```python
from build123d import *

# Parameters (mm, degrees)
ESBO_O1_R                = 7.65
ESBO_O1_R_2              = 1.65
RESSALTO_EXTRUS_O1_DEPTH = 3
FILETE1_R                = 8


with BuildPart() as part:
    # Esboço1 → Ressalto-extrusão1 (new body)
    with BuildSketch(Plane.XY):
        Polygon((-12.827454307, 0), (-5.233177242, 16.48), (5.233177242, 16.48), (12.827454307, 0), (5.233177242, -16.48), (-5.233177242, -16.48), align=None)
        Circle(ESBO_O1_R, mode=Mode.SUBTRACT)
        with Locations((0, -13.5)):
            Circle(ESBO_O1_R_2, mode=Mode.SUBTRACT)
        with Locations((0, 13.5)):
            Circle(ESBO_O1_R_2, mode=Mode.SUBTRACT)
    extrude(amount=RESSALTO_EXTRUS_O1_DEPTH)

    # Filete1
    filete1_edges = [part.edges().sort_by_distance(p)[0] for p in [
        (5.233177242, -16.48, 1.5),
        (-5.233177242, -16.48, 1.5),
        (-12.827454307, 0, 1.5),
        (-5.233177242, 16.48, 1.5),
        (5.233177242, 16.48, 1.5),
        (12.827454307, 0, 1.5),
    ]]
    fillet(filete1_edges, radius=FILETE1_R)


solid = part.part
```
Could you check a few things on this model? Use its own coordinates, in mm. Round coordinates to 2 decimals unless told otherwise and drop trailing zeros. Loops run counter-clockwise (first coordinate to the right, second up) from the corner with the lowest first, then second, coordinate; pieces in that order, holes last. Notation, with made-up numbers: (75.25, 27) - (115.25, 27) arc R26 cw to (115.25, 49) - close; hole circle Ø4 at (54.5, 83). An arc over 180 degrees is marked (long way). Answer as CSV lines item,"result".
1. I want a section at C-C on x = 4. List the corners of the cut face in (y, z) for me, then the cut area to 3 significant figures.
Filled in:
outline,"(-15.47, 0) - (-6.52, 0) - (-6.52, 3) - (-15.47, 3) - close; (6.52, 0) - (15.47, 0) - (15.47, 3) - (6.52, 3) - close"
area,"53.7 mm^2"
2. I want a section at D-D on y = 9. List the corners of the cut face in (x, z) for me, then the cut area to 3 significant figures.
Filled in:
outline,"(-8.68, 0) - (8.68, 0) - (8.68, 3) - (-8.68, 3) - close"
area,"52.1 mm^2"
3. Please list where these lines run through material, in increasing order: line 1 along Y through (x, z) = (0, 0.7); line 2 along Y through (x, z) = (-1.5, 2.85); line 3 along Y through (x, z) = (3, 2.2). Write a range as [from, to].
Filled in:
line 1,"y = [-16.48, -15.15], [-11.85, -7.65], [7.65, 11.85], [15.15, 16.48]"
line 2,"y = [-16.36, -14.19], [-12.81, -7.5], [7.5, 12.81], [14.19, 16.36]"
line 3,"y = [-15.94, -7.04], [7.04, 15.94]"
4. For pin 1 Ø1 at (y, z) = (12.5, 2.5) entering from -X; pin 2 Ø1 at (y, z) = (-11.5, 1) entering from -X, each with a flat end and sliding along its axis, tell me the tip position at first contact or that it passes through.
Filled in:
pin 1,"stops at x = -7.3"
pin 2,"stops at x = -7.76"
5. I want a section at B-B on z = 1.6. List the corners of the cut face in (x, y) for me, then the cut area to 3 significant figures.
Filled in:
outline,"(-11.28, -3.35) - (-7.38, -11.83) arc R8 ccw to (-0.11, -16.48) - (0.11, -16.48) arc R8 ccw to (7.38, -11.83) - (11.28, -3.35) arc R8 ccw to (11.28, 3.35) - (7.38, 11.83) arc R8 ccw to (0.11, 16.48) - (-0.11, 16.48) arc R8 ccw to (-7.38, 11.83) - (-11.28, 3.35) arc R8 ccw to start; hole circle Ø15.3 at (0, 0); hole circle Ø3.3 at (0, -13.5); hole circle Ø3.3 at (0, 13.5)"
area,"372 mm^2"
6. We'd pull the mould along X, two halves only. Please class faces 1 (the face through (-4.48, 15.18, 1.52)), 2 (the face through (-8, 0, 3)), 3 (the face through (-1.658, -7.468, 1.479)), 4 (the face through (12.02, 0.05, 1.52)): +X half, -X half, draft (parallel to the pull), parting line (faces both ways), or undercut.
Filled in:
face 1,"-X half"
face 2,"draft"
face 3,"undercut"
face 4,"+X half"
7. I want a section at A-A on y = 14. List the corners of the cut face in (x, z) for me.
Filled in:
outline,"(-5.9, 0) - (-1.57, 0) - (-1.57, 3) - (-5.9, 3) - close; (1.57, 0) - (5.9, 0) - (5.9, 3) - (1.57, 3) - close"
